Source: three-view drawing plus pictorial views. Frame: mm from the lowest corner of the part. A direction names the side the tool comes from. Coordinates: 2 decimals unless noted, no trailing zeros. Write each loop counter-clockwise with the first axis right and the second up, starting at its lowest first coordinate (ties: lowest second). Pieces come first, ordered by that corner, then holes. Notation, with made-up numbers: (79.5, 67.25) -> (120.5, 67.25) arc R12 cw to (120.5, 89.25) -> close; hole circle Ø5 at (19, 3.5). An arc over 180 degrees is marked (long way). One line per item, written item: value. Start each with the question number.
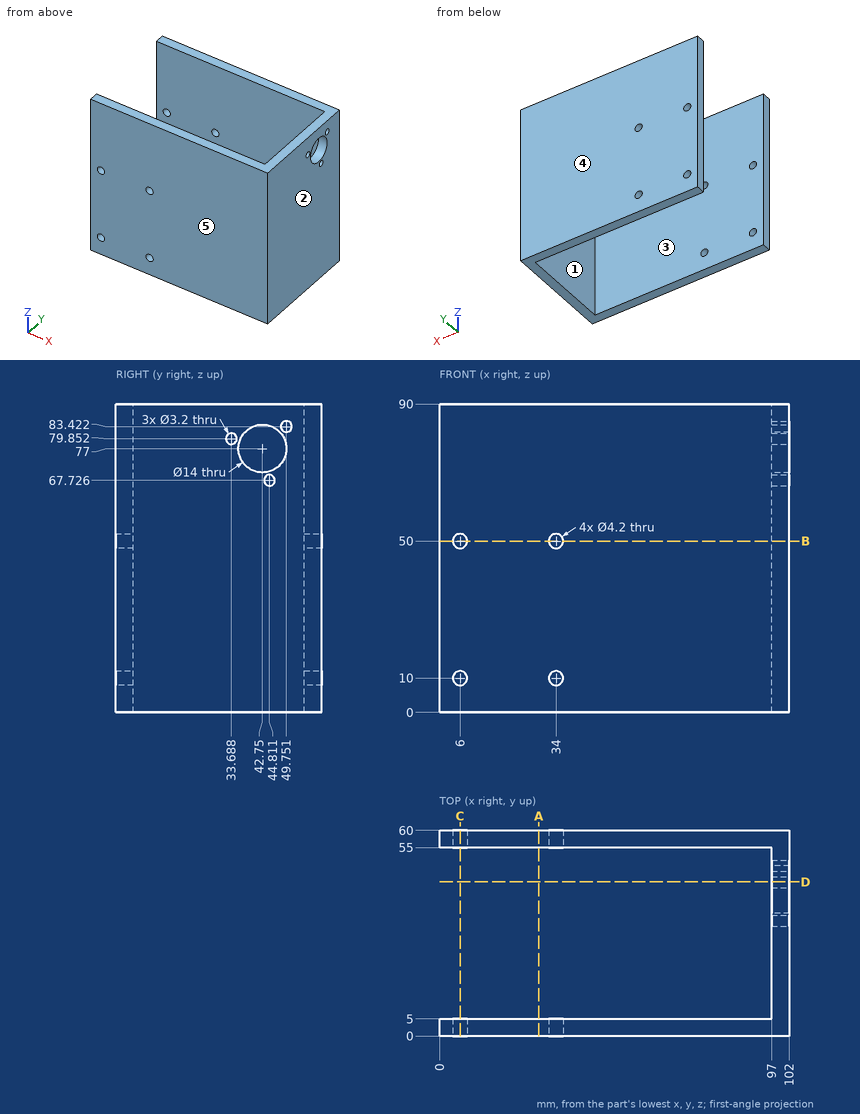
Q1. Cut plane C-C on x = 6. Output: boundary loops of the cut face in (y, z).
Q2. Draft query along Y for the marked faces 3, 4 and 5. Return one class per face: pulls with the +Y half, pulls with the -Y half, needs draft (parallel to the pull), parting line crosses it, or undercut.
Q3. Cut plane A-A on x = 29. Output: boundary loops of the cut face in (y, z).
Q4. Cut plane D-D on y = 45. Output: boundary loops of the cut face in (x, z) (1 decimal), and give its area (3 significant figures).
Q5. First-contact query: P1, Ø16, axis at y = 42.75, z = 77, coming from the -X side; P2, Ø5, axis at x = 6, z = 10, coming from the -Y side. Flat tips, straight axial feed; report the tip coordinate or a pass-through.
Q6. Line query: L1, parallel to X at y = 57.05, z = 50; L2, parallel to Y at x = 46, z = 12; L3, parallel to Z at x = 34, y = 57.8. Output: solid intervals per line, ascending. Write a range as from..to.
Q7. Access query for the marked faces 1 and 2. Directions: +Z, -Z, +X, -X, +Y, -Y. A direction counts if a zero-diameter tool reaches every point of the face in a straight line with its end or side. Return the directions, or none.
Q8. Cut plane B-B on z = 50. Output: boundary loops of the cut face in (x, y).
Solution:
1. outline: (0, 0) -> (5, 0) -> (5, 7.9) -> (0, 7.9) -> close; (0, 12.1) -> (5, 12.1) -> (5, 47.9) -> (0, 47.9) -> close; (0, 52.1) -> (5, 52.1) -> (5, 90) -> (0, 90) -> close; (55, 0) -> (60, 0) -> (60, 7.9) -> (55, 7.9) -> close; (55, 12.1) -> (60, 12.1) -> (60, 47.9) -> (55, 47.9) -> close; (55, 52.1) -> (60, 52.1) -> (60, 90) -> (55, 90) -> close
2. face 3: undercut
2. face 4: pulls with the +Y half
2. face 5: pulls with the -Y half
3. outline: (0, 0) -> (5, 0) -> (5, 90) -> (0, 90) -> close; (55, 0) -> (60, 0) -> (60, 90) -> (55, 90) -> close
4. outline: (97, 0) -> (102, 0) -> (102, 66.1) -> (97, 66.1) -> close; (97, 69.3) -> (102, 69.3) -> (102, 70.4) -> (97, 70.4) -> close; (97, 83.6) -> (102, 83.6) -> (102, 90) -> (97, 90) -> close
4. area: 368 mm²
5. P1: x = 97
5. P2: y = 0
6. L1: 0..3.9, 8.1..31.9, 36.1..102
6. L2: 0..5, 55..60
6. L3: 0..7.9, 12.1..47.9, 52.1..90
7. face 1: +Z, -Z, -X
7. face 2: +Z, -Z, +X, +Y, -Y
8. outline: (0, 0) -> (3.9, 0) -> (3.9, 5) -> (0, 5) -> close; (0, 55) -> (3.9, 55) -> (3.9, 60) -> (0, 60) -> close; (8.1, 0) -> (31.9, 0) -> (31.9, 5) -> (8.1, 5) -> close; (8.1, 55) -> (31.9, 55) -> (31.9, 60) -> (8.1, 60) -> close; (36.1, 0) -> (102, 0) -> (102, 60) -> (36.1, 60) -> (36.1, 55) -> (97, 55) -> (97, 5) -> (36.1, 5) -> close
